The model under review builds one solid part; all positions refer to its coordinate system, in mm. A direction names the side the tool comes from. Round coordinates to 2 decimals unless told otherwise and drop trailing zeros. Write each loop counter-clockwise with the first axis right and the second up, starting at its lowest first coordinate (ties: lowest second). Pieces come first, ordered by that corner, then holes. Notation, with made-up numbers: (-6, 82) -> (4, 82) arc R26 ccw to (4, 112) -> close; hole circle Ø2 at (-31, -26). An arc over 180 degrees is marked (long way). Return JSON: item names as keys, results as strings. Group by question number.
1. Take a section at B-B, the plane x = -88.5. Write out the cut boundary in (y, z) (3 decimals), then the cut area to 3 significant figures.
2. Take a section at C-C, the plane y = 27.5. Write out the cut boundary in (x, z) (3 decimals), then the cut area to 3 significant figures.
3. For line 1 along Y through (x, z) = (-84, 0.75); line 2 along X through (y, z) = (-7, 0.3); line 3 along Y through (x, z) = (-78, 1.25), list the stretches that pass through material, from the lowest coordinate up. Write a range as from..to.
4. Tool access review of faces 1 (the flat face through (-58, 0, 2)), 2 (the flat face through (-68, 3.221, 2)), 3 (the flat face through (-67, -19.05, 2)): name each direction out of +Z, -Z, +X, -X, +Y, -Y from which nothing blocks a thin tool from reaching the whole face with its end or side.
5. Take a section at D-D, the plane x = -100. Write out the cut boundary in (y, z) (3 decimals).
6. Clearance check with flat-ended pins moving along their axes: P1, Ø1.6, axis at x = -60, y = 0, coming from the -Z side; P2, Ø1.6, axis at y = -13, z = 2, coming from the -X side; P3, Ø4.5, axis at x = -99.59, y = 43.76, coming from the -Z side; P4, Ø1, axis at y = -13.5, z = 1, coming from the +X side. State where each tip first meets the part, or that it passes through.
7. Mouldability with a two-part tool opening along Y and no side actions: class faces 4 (the cylindrical face through (-81.48, 3.74, 1.57)), 5 (the flat face through (-80, 0, 2)), 6 (the flat face through (-75, -10, 2)) as pulls with the +Y half, pulls with the -Y half, needs draft (parallel to the pull), parting line crosses it, or undercut.
8. Take a section at A-A, the plane y = 50.5. Write out the cut boundary in (x, z) (3 decimals), then the cut area to 3 significant figures.
from build123d import *

# Parameters (mm, degrees)
SKETCH1_R           = 8
SKETCH1_R_2         = 1.89865
SKETCH1_R_3         = 1.9939
BOSS_EXTRUDE1_DEPTH = 3.175
FILLET1_R           = 10
SKETCH2_W           = 15
SKETCH2_H           = 19.05
BOSS_EXTRUDE2_DEPTH = 3.175
SKETCH3_R           = 1
CUT_EXTRUDE1_DEPTH  = 158.949594679
CHAMFER1_SIZE       = 1
FILLET2_R           = 1
SKETCH4_W           = 7.99338
SKETCH4_H           = 3.22072
CUT_EXTRUDE2_DEPTH  = 158.949594679
CUT_EXTRUDE3_DEPTH  = 158.949594679
FILLET3_R           = 10
SKETCH6_R           = 1
CUT_EXTRUDE4_DEPTH  = 124.748935267
FILLET4_R           = 1


with BuildPart() as part:
    # Sketch1 → Boss-Extrude1 (new body)
    with BuildSketch(Plane.XY):
        with BuildLine():
            Line((-40.498784978, 0), (0, 0))
            Line((0, 0), (0, 75))
            ThreePointArc((0, 75), (-37.5, 112.5), (-75, 75))
            Line((-75, 75), (-75, 55))
            Line((-75, 55), (-83.323029145, 55))
            ThreePointArc((-83.323029145, 55), (-110.823029145, 27.5), (-83.323029145, 0))
            Line((-83.323029145, 0), (-40.498784978, 0))
        make_face()
        with Locations((-83.323029145, 27.5)):
            Circle(SKETCH1_R, mode=Mode.SUBTRACT)
        with Locations((-67.059573177, 11.236544033)):
            Circle(SKETCH1_R_2, mode=Mode.SUBTRACT)
        with Locations((-83.323029145, 50.5)):
            Circle(SKETCH1_R_3, mode=Mode.SUBTRACT)
        with Locations((-99.586485112, 11.236544033)):
            Circle(SKETCH1_R_2, mode=Mode.SUBTRACT)
        with Locations((-60.323029145, 27.5)):
            Circle(SKETCH1_R_3, mode=Mode.SUBTRACT)
        with Locations((-99.586485112, 43.763455967)):
            Circle(SKETCH1_R_2, mode=Mode.SUBTRACT)
        with Locations((-83.323029145, 4.5)):
            Circle(SKETCH1_R_3, mode=Mode.SUBTRACT)
        with Locations((-106.323029145, 27.5)):
            Circle(SKETCH1_R_3, mode=Mode.SUBTRACT)
    extrude(amount=BOSS_EXTRUDE1_DEPTH)

    # Fillet1
    fillet1_edges = [part.edges().sort_by_distance(p)[0] for p in [
        (-75, 55, 1.5875),
    ]]
    fillet(fillet1_edges, radius=FILLET1_R)

    # Sketch2 → Boss-Extrude2 (add)
    with BuildSketch(Plane(origin=(0, 0, 0), x_dir=(-1, 0, 0), z_dir=(0, 0, -1))):
        with Locations((7.5, -9.525)):
            Rectangle(SKETCH2_W, SKETCH2_H)
        with Locations((37.5, -9.525)):
            Rectangle(SKETCH2_W, SKETCH2_H)
        with Locations((67.5, -9.525)):
            Rectangle(SKETCH2_W, SKETCH2_H)
    extrude(amount=-BOSS_EXTRUDE2_DEPTH)

    # Sketch3 → Cut-Extrude1 (cut, through all)
    with BuildSketch(Plane.XY.offset(3.175)):
        with Locations((-75, 0)):
            Circle(SKETCH3_R)
        with Locations((-60, 0)):
            Circle(SKETCH3_R)
        with Locations((-45, 0)):
            Circle(SKETCH3_R)
        with Locations((-30, 0)):
            Circle(SKETCH3_R)
        with Locations((-15, 0)):
            Circle(SKETCH3_R)
    extrude(amount=-CUT_EXTRUDE1_DEPTH, mode=Mode.SUBTRACT)

    # Chamfer1
    chamfer1_edges = [part.edges().sort_by_distance(p)[0] for p in [
        (0, -19.05, 1.5875),
        (-15, -19.05, 1.5875),
        (-30, -19.05, 1.5875),
        (-45, -19.05, 1.5875),
        (-60, -19.05, 1.5875),
        (-75, -19.05, 1.5875),
    ]]
    chamfer(chamfer1_edges, length=CHAMFER1_SIZE)

    # Fillet2
    fillet2_edges = [part.edges().sort_by_distance(p)[0] for p in [
        (-75, -1, 1.5875),
        (-76, 0, 1.5875),
        (-60, -1, 1.5875),
        (-59, 0, 1.5875),
        (-45, -1, 1.5875),
        (-46, 0, 1.5875),
        (-30, -1, 1.5875),
        (-29, 0, 1.5875),
        (-15, -1, 1.5875),
        (-16, 0, 1.5875),
    ]]
    fillet(fillet2_edges, radius=FILLET2_R)

    # Sketch4 → Cut-Extrude2 (cut, through all)
    with BuildSketch(Plane.XY.offset(3.175)):
        with Locations((-67.5, 1.61036)):
            Rectangle(SKETCH4_W, SKETCH4_H)
    extrude(amount=-CUT_EXTRUDE2_DEPTH, mode=Mode.SUBTRACT)

    # Sketch5 → Cut-Extrude3 (cut, through all)
    with BuildSketch(Plane(origin=(0, 0, 0), x_dir=(-1, 0, 0), z_dir=(0, 0, -1))):
        Polygon((84.552807772, 54.972488867), (46.732050808, 54.972488867), (46.732050808, 0), (46.732050808, -19.05), (0, -19.05), (0, 112.5), (84.552807772, 112.5), align=None)
    extrude(amount=-CUT_EXTRUDE3_DEPTH, mode=Mode.SUBTRACT)

    # Fillet3
    fillet3_edges = [part.edges().sort_by_distance(p)[0] for p in [
        (-46.732050808, 0, 1.5875),
        (-46.732050808, 54.972488867, 1.5875),
    ]]
    fillet(fillet3_edges, radius=FILLET3_R)

    # Sketch6 → Cut-Extrude4 (cut, through all)
    with BuildSketch(Plane(origin=(0, 0, 0), x_dir=(-1, 0, 0), z_dir=(0, 0, -1))):
        with Locations((63.50331, 3.22072)):
            Circle(SKETCH6_R)
        with Locations((71.49669, 3.22072)):
            Circle(SKETCH6_R)
        with Locations((71.49669, 0)):
            Circle(SKETCH6_R)
        with Locations((63.50331, 0)):
            Circle(SKETCH6_R)
    extrude(amount=-CUT_EXTRUDE4_DEPTH, mode=Mode.SUBTRACT)

    # Fillet4
    # the kernel refuses this fillet: 1 mm, written as the material it takes off along each edge
    with BuildSketch(Plane(origin=(-70.49669, 3.22072, 5.005127019), x_dir=(1, 0, 0), z_dir=(0, 0, -1)), Plane(origin=(-71.49669, 1, 5.005127019), x_dir=(0, 1, 0), z_dir=(0, 0, -1)), Plane(origin=(-63.50331, 2.22072, 5.005127019), x_dir=(0, -1, 0), z_dir=(0, 0, -1))) as fillet4_piece_1:
        with BuildLine():
            CenterArc((0.732050808, -1), FILLET4_R, 90, 60)
            ThreePointArc((-0.133974596, -0.5), (-0.034074174, -0.258819045), (0, 0))
            Line((0, 0), (0.732050808, 0))
        make_face()
    extrude(amount=6.835254038, mode=Mode.SUBTRACT)
    with BuildSketch(Plane(origin=(-71.49669, 2.22072, 5.005127019), x_dir=(-0.9659258262890673, 0.25881904510252446, 0), z_dir=(0, 0, -1)), Plane(origin=(-70.49669, 0, 5.005127019), x_dir=(-0.25881904510253056, -0.9659258262890658, 0), z_dir=(0, 0, -1))) as fillet4_piece_2:
        with BuildLine():
            CenterArc((0.776457135, -0.965925826), FILLET4_R, 105, 60)
            Line((-0.189468691, -0.707106781), (0, 0))
            ThreePointArc((0, 0), (0.258819045, -0.034074174), (0.51763809, 0))
        make_face()
    extrude(amount=6.835254038, mode=Mode.SUBTRACT)
    with BuildSketch(Plane(origin=(-64.50331, 0, -1.830127019), x_dir=(-1, 0, 0), z_dir=(0, 0, 1)), Plane(origin=(-63.50331, 1, 5.005127019), x_dir=(0, 1, 0), z_dir=(0, 0, -1))) as fillet4_piece_3:
        with BuildLine():
            CenterArc((0.732050808, 1), FILLET4_R, 210, 60)
            ThreePointArc((-0.133974596, 0.5), (-0.034074174, 0.258819045), (0, 0))
            Line((0, 0), (0.732050808, 0))
        make_face()
    extrude(amount=6.835254038, mode=Mode.SUBTRACT)
    with BuildSketch(Plane(origin=(-64.50331, 3.22072, -1.830127019), x_dir=(0.25881904510250514, 0.9659258262890725, 0), z_dir=(0, 0, 1))) as fillet4_piece_4:
        with BuildLine():
            CenterArc((0.776457135, 0.965925826), FILLET4_R, 195, 60)
            Line((-0.189468691, 0.707106781), (0, 0))
            ThreePointArc((0, 0), (0.258819045, 0.034074174), (0.51763809, 0))
        make_face()
    extrude(amount=6.835254038, mode=Mode.SUBTRACT)


solid = part.part
Output:
{
 "1": {"outline": "(0.492, 0) -> (21.401, 0) -> (21.401, 3.175) -> (0.492, 3.175) -> close; (33.599, 0) -> (54.508, 0) -> (54.508, 3.175) -> (33.599, 3.175) -> close", "area": "133 mm^2"},
 "2": {"outline": "(-110.823, 0) -> (-108.317, 0) -> (-108.317, 3.175) -> (-110.823, 3.175) -> close; (-104.329, 0) -> (-91.323, 0) -> (-91.323, 3.175) -> (-104.329, 3.175) -> close; (-75.323, 0) -> (-62.317, 0) -> (-62.317, 3.175) -> (-75.323, 3.175) -> close; (-58.329, 0) -> (-46.732, 0) -> (-46.732, 3.175) -> (-58.329, 3.175) -> close", "area": "127 mm^2"},
 "3": {"line 1": "y = 0.01..2.62, 6.38..19.53, 35.47..48.62, 52.38..54.97", "line 2": "x = -75..-60", "line 3": "y = 0..21.53, 33.47..54.97"},
 "4": {"face 1": "+Z, -Z, +X, -Y", "face 2": "+Z, -Z", "face 3": "+Z, -Z, +X, -X, -Y"},
 "5": {"outline": "(5.634, 0) -> (9.383, 0) -> (9.383, 3.175) -> (5.634, 3.175) -> close; (13.09, 0) -> (41.91, 0) -> (41.91, 3.175) -> (13.09, 3.175) -> close; (45.617, 0) -> (49.366, 0) -> (49.366, 3.175) -> (45.617, 3.175) -> close"},
 "6": {"P1": "passes through", "P2": "stops at x = -75", "P3": "stops at z = 0", "P4": "stops at x = -60"},
 "7": {"face 4": "undercut", "face 5": "pulls with the -Y half", "face 6": "needs draft"},
 "8": {"outline": "(-98.398, 0) -> (-85.317, 0) -> (-85.317, 3.175) -> (-98.398, 3.175) -> close; (-81.329, 0) -> (-48.399, 0) -> (-48.399, 3.175) -> (-81.329, 3.175) -> close", "area": "146 mm^2"}
}
